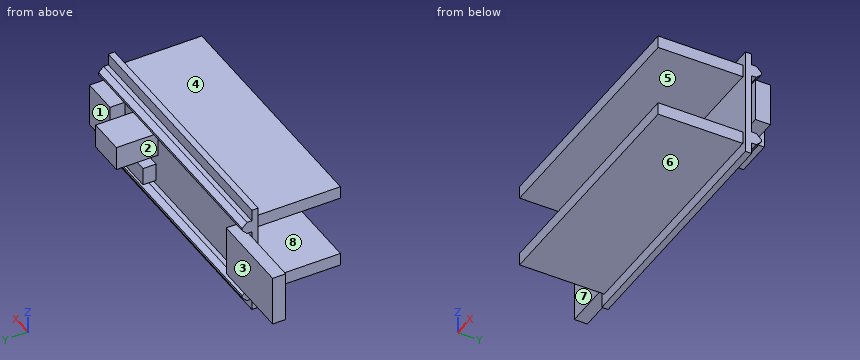
```python
from build123d import *

# Parameters (mm, degrees)
SKETCH_2_W      = 52.6
SKETCH_2_H      = 22.6
EXTRUDE_1_DEPTH = 1.3
SKETCH_3_W      = 52.6
SKETCH_3_H      = 2.5
EXTRUDE_2_DEPTH = 2
CHAMFER_1_SIZE  = 1
SKETCH_4_W      = 6.1
SKETCH_4_H      = 9
SKETCH_4_W_2    = 1.4
EXTRUDE_3_DEPTH = 3.1
SKETCH_5_W      = 12.4
SKETCH_5_H      = 10.4
SKETCH_5_W_2    = 4.6
EXTRUDE_4_DEPTH = 2.7
SKETCH_6_W      = 7.6
SKETCH_6_H      = 5
EXTRUDE_5_DEPTH = 8.6
SKETCH_7_W      = 6
SKETCH_7_H      = 3.7
EXTRUDE_6_DEPTH = 2.7
SKETCH_8_W      = 50.8
SKETCH_8_H      = 2.6
EXTRUDE_8_DEPTH = 17.5


with BuildPart() as part:
    # 草图2 → 凸台-拉伸1 (new body)
    with BuildSketch(Plane(origin=(0, 0, 0), x_dir=(1, 0, 0), z_dir=(0, 1, 0))):
        Rectangle(SKETCH_2_W, SKETCH_2_H)
    extrude(amount=EXTRUDE_1_DEPTH)

    # 草图3 → 凸台-拉伸2 (add)
    with BuildSketch(Plane(origin=(0, 1.3, 0), x_dir=(1, 0, 0), z_dir=(0, 1, 0))):
        with Locations((0, 7.65)):
            Rectangle(SKETCH_3_W, SKETCH_3_H)
        with Locations((0, -7.65)):
            Rectangle(SKETCH_3_W, SKETCH_3_H)
    extrude(amount=EXTRUDE_2_DEPTH)

    # 倒角1
    chamfer_1_edges = [part.edges().sort_by_distance(p)[0] for p in [
        (0, 3.3, -8.9),
        (0, 3.3, -6.4),
        (0, 3.3, 6.4),
        (0, 3.3, 8.9),
    ]]
    chamfer(chamfer_1_edges, length=CHAMFER_1_SIZE)

    # 草图4 → 凸台-拉伸3 (add)
    with BuildSketch(Plane(origin=(0, 1.3, 0), x_dir=(1, 0, 0), z_dir=(0, 1, 0))):
        with Locations((23.25, 0)):
            Rectangle(SKETCH_4_W, SKETCH_4_H)
        with Locations((27, 0)):
            Rectangle(SKETCH_4_W_2, SKETCH_4_H)
    extrude(amount=EXTRUDE_3_DEPTH)

    # 草图5 → 凸台-拉伸4 (add)
    with BuildSketch(Plane(origin=(0, 1.3, 0), x_dir=(1, 0, 0), z_dir=(0, 1, 0))):
        with Locations((-32.5, 0)):
            Rectangle(SKETCH_5_W, SKETCH_5_H)
        with Locations((-24, 0)):
            Rectangle(SKETCH_5_W_2, SKETCH_5_H)
    extrude(amount=EXTRUDE_4_DEPTH)

    # 草图6 → 凸台-拉伸5 (add)
    with BuildSketch(Plane(origin=(0, 1.3, 0), x_dir=(1, 0, 0), z_dir=(0, 1, 0))):
        with Locations((11.9, -3.1)):
            Rectangle(SKETCH_6_W, SKETCH_6_H)
    extrude(amount=EXTRUDE_5_DEPTH)

    # 草图7 → 凸台-拉伸6 (add)
    with BuildSketch(Plane(origin=(0, 1.3, 0), x_dir=(1, 0, 0), z_dir=(0, 1, 0))):
        with Locations((11.8, 3.735961984)):
            Rectangle(SKETCH_7_W, SKETCH_7_H)
    extrude(amount=EXTRUDE_6_DEPTH)

    # 草图8 → 凸台-拉伸8 (add)
    with BuildSketch(Plane.XZ):
        with Locations((0, -7.6)):
            Rectangle(SKETCH_8_W, SKETCH_8_H)
        with Locations((0, 7.6)):
            Rectangle(SKETCH_8_W, SKETCH_8_H)
    extrude(amount=EXTRUDE_8_DEPTH)


solid = part.part
```
Verification items for the finished model (mm, model axes). Face numbers are marked on the shaded views. A direction names the side the tool comes from. Round coordinates to 2 decimals unless told otherwise and drop trailing zeros. Write each loop counter-clockwise with the first axis right and the second up, starting at its lowest first coordinate (ties: lowest second). Pieces come first, ordered by that corner, then holes. Notation, with made-up numbers: (60.5, 85.25) - (78.5, 85.25) arc R12 cw to (78.5, 97.25) - close; hole circle Ø6 at (66, 44). An arc over 180 degrees is marked (long way). Answer as a JSON object with one key per item and string values. Group by question number.
Q1. Thickness scan on line 1 (Z direction, x = 17.5, y = -2.75); line 2 (Y direction, x = 2, z = -5); line 3 (Y direction, x = -4.5, z = 7.5). Record the ranges inside material, lowest first.
Q2. Section check A-A, the plane x = -23.5. Enter the section's corners in (y, z), plus the area to 3 significant figures.
Q3. Go/stop test with flat-tipped pins: pin 1 Ø9 at (x, y) = (2.5, -9.5) entering from +Z; pin 2 Ø3 at (x, z) = (12, -3.5) entering from +Y; pin 3 Ø1.3 at (y, z) = (-8.5, 7.5) entering from -X. Record where each tip stops, or that it passes through.
Q4. Mould release check, pull along Z, two halves, no side actions. Record for the marked faces 6, 7 and 8: released by +Z, released by -Z, zero draft, split by the parting line, or undercut.
Q5. Section check C-C, the plane z = -2.5. Enter the section's corners in (x, y), plus the area to 3 significant figures.
Q6. Section check B-B, the plane y = -7. Enter the section's corners in (x, z).
Q7. Tool access check on the marked faces 1, 2, 3, 4 and 5. Record the directions out of +Z, -Z, +X, -X, +Y, -Y that give a thin tool (end or side, any length) a straight path to the whole face; none if there is none.
Q8. Section check D-D, the plane y = 8. Enter the section's corners in (x, z), plus the area to 3 significant figures.
Found:
{
 "1": {"line 1": "z = -8.9 to -6.3, 6.3 to 8.9", "line 2": "y = 0 to 1.3", "line 3": "y = -17.5 to 3.3"},
 "2": {"outline": "(-17.5, -8.9) - (0, -8.9) - (0, -11.3) - (1.3, -11.3) - (1.3, -8.9) - (2.3, -8.9) - (3.3, -7.9) - (3.3, -7.4) - (2.3, -6.4) - (1.3, -6.4) - (1.3, -5.2) - (4, -5.2) - (4, 5.2) - (1.3, 5.2) - (1.3, 6.4) - (2.3, 6.4) - (3.3, 7.4) - (3.3, 7.9) - (2.3, 8.9) - (1.3, 8.9) - (1.3, 11.3) - (0, 11.3) - (0, 8.9) - (-17.5, 8.9) - (-17.5, 6.3) - (0, 6.3) - (0, -6.3) - (-17.5, -6.3) - close", "area": "156 mm^2"},
 "3": {"pin 1": "stops at z = 8.9", "pin 2": "stops at y = 4", "pin 3": "stops at x = -25.4"},
 "4": {"face 6": "released by -Z", "face 7": "zero draft", "face 8": "undercut"},
 "5": {"outline": "(-38.7, 1.3) - (-26.3, 1.3) - (-26.3, 0) - (26.3, 0) - (26.3, 1.3) - (27.7, 1.3) - (27.7, 4.4) - (20.2, 4.4) - (20.2, 1.3) - (14.8, 1.3) - (14.8, 4) - (8.8, 4) - (8.8, 1.3) - (-21.7, 1.3) - (-21.7, 4) - (-38.7, 4) - close", "area": "154 mm^2"},
 "6": {"outline": "(-25.4, -8.9) - (25.4, -8.9) - (25.4, -6.3) - (-25.4, -6.3) - close; (-25.4, 6.3) - (25.4, 6.3) - (25.4, 8.9) - (-25.4, 8.9) - close"},
 "7": {"face 1": "+Z, -Z, +X, +Y", "face 2": "+Y", "face 3": "+Z, -Z, -X, +Y", "face 4": "+Z, +X, -X, -Y", "face 5": "+X, -X, -Y"},
 "8": {"outline": "(8.1, 0.6) - (15.7, 0.6) - (15.7, 5.6) - (8.1, 5.6) - close", "area": "38.0 mm^2"}
}
